from build123d import *

# Parameters (mm, degrees)
SKETCH_4_W          = 36.75
SKETCH_4_H          = 10
EXTRUDE_1_DEPTH     = 5
EXTRUDE_START       = 5
SKETCH_4_3_W        = 5
SKETCH_4_3_H        = 10
EXTRUDE_2_DEPTH     = 8
SKETCH_5_W          = 5
SKETCH_5_H          = 13
EXTRUDE_3_DEPTH     = 8
SKETCH_6_R          = 1.5
SKETCH_6_W          = 8
SKETCH_6_H          = 5
CUT_EXTRUDE_1_DEPTH = 39.74354785
SKETCH_6_3_R        = 2.25
CUT_EXTRUDE_2_DEPTH = 2
SKETCH_7_R          = 2.25
CUT_EXTRUDE_3_DEPTH = 2
SKETCH_7_3_R        = 1.5
CUT_EXTRUDE_4_DEPTH = 42.696072957
FILLET_1_R          = 4


with BuildPart() as part:
    # 草图4 → 凸台-拉伸1 (new body)
    with BuildSketch(Plane(origin=(0, 0, 0), x_dir=(1, 0, 0), z_dir=(0, 1, 0))):
        with Locations((-18.375, -5)):
            Rectangle(SKETCH_4_W, SKETCH_4_H)
    extrude(amount=EXTRUDE_1_DEPTH)

    # 草图4<3> → 凸台-拉伸2 (add)
    with BuildSketch(Plane(origin=(0, 0, 0), x_dir=(1, 0, 0), z_dir=(0, 1, 0)).offset(EXTRUDE_START)):
        with Locations((-2.5, -5)):
            Rectangle(SKETCH_4_3_W, SKETCH_4_3_H)
    extrude(amount=EXTRUDE_2_DEPTH)

    # 草图5 → 凸台-拉伸3 (add)
    with BuildSketch(Plane.XY.offset(10)):
        with Locations((-2.5, 6.5)):
            Rectangle(SKETCH_5_W, SKETCH_5_H)
    extrude(amount=EXTRUDE_3_DEPTH)

    # 草图6 → 切除-拉伸1 (cut, through all)
    with BuildSketch(Plane.ZY.offset(5)):
        with Locations((5, 9)):
            Circle(SKETCH_6_R)
        with Locations((14, 4)):
            Circle(SKETCH_6_R)
        with Locations((14, 10.5)):
            Rectangle(SKETCH_6_W, SKETCH_6_H)
    extrude(amount=-CUT_EXTRUDE_1_DEPTH, mode=Mode.SUBTRACT)

    # 草图6<3> → 切除-拉伸2 (cut)
    with BuildSketch(Plane.ZY.offset(5)):
        with Locations((5, 9)):
            Circle(SKETCH_6_3_R)
        with Locations((14, 4)):
            Circle(SKETCH_6_3_R)
    extrude(amount=-CUT_EXTRUDE_2_DEPTH, mode=Mode.SUBTRACT)

    # 草图7 → 切除-拉伸3 (cut)
    with BuildSketch(Plane(origin=(0, 5, 0), x_dir=(1, 0, 0), z_dir=(0, 1, 0))):
        with Locations(Location((-31.75, -5, 0), (0, 0, 270))):
            Circle(SKETCH_7_R)
        with Locations(Location((-10, -5, 0), (0, 0, 270))):
            Circle(SKETCH_7_R)
    extrude(amount=-CUT_EXTRUDE_3_DEPTH, mode=Mode.SUBTRACT)

    # 草图7<3> → 切除-拉伸4 (cut, through all)
    with BuildSketch(Plane(origin=(0, 5, 0), x_dir=(1, 0, 0), z_dir=(0, 1, 0))):
        with Locations(Location((-31.75, -5, 0), (0, 0, 270))):
            Circle(SKETCH_7_3_R)
        with Locations(Location((-10, -5, 0), (0, 0, 270))):
            Circle(SKETCH_7_3_R)
    extrude(amount=-CUT_EXTRUDE_4_DEPTH, mode=Mode.SUBTRACT)

    # 圆角1
    fillet_1_edges = [part.edges().sort_by_distance(p)[0] for p in [
        (-2.5, 13, 10),
        (-2.5, 0, 18),
        (-2.5, 8, 18),
    ]]
    fillet(fillet_1_edges, radius=FILLET_1_R - 0.0001)  # a hair under: the kernel refuses the full size


solid = part.part
Part model, mm, in its own coordinate system. A direction names the side the tool comes from. Round coordinates to 2 decimals unless told otherwise and drop trailing zeros. Order: outer loops, then holes, each group sorted by start corner. A loop starts at its lowest first (then second) coordinate and runs counter-clockwise, first axis right, second up. Notation, with made-up numbers: (79.5, 39) -> (113.5, 39) arc R15 ccw to (113.5, 54) -> close; hole circle Ø4 at (20, -22.5). An arc over 180 degrees is marked (long way). Put each result on its own line as item: value.
Q1. Band-saw the part on D-D (z = 2). Give the cut face in (x, y).
From the geometry:
outline: (-36.75, 0) -> (0, 0) -> (0, 13) -> (-5, 13) -> (-5, 5) -> (-36.75, 5) -> close
Q2. Band-saw the part on A-A (x = -10). Give the cut face in (y, z).
From the geometry:
outline: (0, 0) -> (5, 0) -> (5, 2.75) -> (3, 2.75) -> (3, 3.5) -> (0, 3.5) -> close; (0, 6.5) -> (3, 6.5) -> (3, 7.25) -> (5, 7.25) -> (5, 10) -> (0, 10) -> close
Q3. Pull direction X, two halves, no side cores. Call faces 6 (the face through (0, 5, 7)), 7 (the face through (-1.52, 4.07, 12.5)), 8 (the face through (-11.33, 1.52, 5.69)), 9 (the face through (-29.853, 4.014, 6.21)): pulls with the +X half, pulls with the -X half, needs draft (parallel to the pull), parting line crosses it, or undercut.
From the geometry:
face 6: pulls with the +X half
face 7: needs draft
face 8: undercut
face 9: undercut
Q4. Tool access for faces 1 (the face through (-10, 3, 3)), 2 (the face through (-4.014, 4.676, 16.146)), 3 (the face through (-21, 5, 5)), 4 (the face through (-2.5, 8.5, 10)), 5 (the face through (-5, 6, 9)): list every direction of +Z, -Z, +X, -X, +Y, -Y with a clear straight run to the whole face (end or side of a thin tool).
From the geometry:
face 1: +Y
face 2: -X
face 3: +Z, -Z, -X, +Y
face 4: +Z, +X, -X, +Y
face 5: +Z, -X, +Y
Q5. Pin check, flat tips, straight feed: pin 1 Ø6 at (x, z) = (-31.75, 5) entering from +Y; pin 2 Ø0.5 at (x, y) = (-2, 8.5) entering from +Z; pin 3 Ø1.3 at (x, z) = (-31, 5.5) entering from +Y. Stop position of each tip, or through.
From the geometry:
pin 1: stops at y = 5
pin 2: stops at z = 10
pin 3: stops at y = 3
Q6. Band-saw the part on B-B (z = 5). State how many separate pieces and enclosed holes the cut face has, and give its area (3 significant figures).
From the geometry:
separate pieces: 4
enclosed holes: 0
area: 170 mm2
Q7. Wall check: line 1 (Y direction, x = -0.8, z = 5); line 2 (X direction, y = 3.75, z = 3); line 3 (Y direction, x = -3.8, z = 5). Give the ranges that are in metal, low to high. Write a range as [from, to].
From the geometry:
line 1: y = [0, 7.5], [10.5, 13]
line 2: x = [-36.75, -32.78], [-30.72, -11.03], [-8.97, 0]
line 3: y = [0, 6.75], [11.25, 13]
